For this review, take the finished solid that the model builds, in its own axes (mm). A direction names the side the tool comes from. Round coordinates to 2 decimals unless told otherwise and drop trailing zeros. Loops run counter-clockwise (first coordinate to the right, second up) from the corner with the lowest first, then second, coordinate; pieces in that order, holes last.
1) Mouldability with a two-part tool opening along Y and no side actions: class faces 4 (the flat face through (21.3, 4, 9)), 5 (the flat face through (29, 18, 6)), 6 (the flat face through (-3, -6, 5)), 7 (the flat face through (-3, 15, 1)) as pulls with the +Y half, pulls with the -Y half, needs draft (parallel to the pull), parting line crosses it, or undercut.
2) Tool access review of faces 1 (the flat face through (32.5, 3, 9)), 2 (the flat face through (23, 5, -2)), 3 (the flat face through (-5, 6, 5)): name each direction out of +Z, -Z, +X, -X, +Y, -Y from which nothing blocks a thin tool from reaching the whole face with its end or side.
3) Take a section at B-B (z = 8.75). State the section outline as (x, y) points.
4) Take a section at C-C (z = 4). State the section outline as (x, y) points, then the cut area to 3 significant figures.
5) Take a section at A-A (y = 7). State the section outline as (x, z) points (3 decimals), then the cut area to 3 significant figures.
6) Wall thickness on L1, parallel to X at y = 3.25, z = 0; L2, parallel to X at y = 15.5, z = 3.25; L3, parallel to Y at x = 32, z = 8.25: over which ranges is each line inside the solid? List them lowest first.
7) Take a section at D-D (y = 10). State the section outline as (x, z) points (3 decimals).
8) Insertion check: pin 1 (6 mm diameter, centred on x = 22.5, y = 4.5, fed in from -Z); pin 2 (0.5 mm diameter, centred on y = 2, z = 9, fed in from -X); pin 3 (4.5 mm diameter, centred on x = 36.5, z = -3, fed in from -Y); pin 4 (5.5 mm diameter, centred on x = 28, y = 6.5, fed in from +Z). Each pin has a flat end and moves straight along its axis. Give the tip position at first contact, or say it passes through.
Autodesk Fusion 360 part; units mm, degrees
sketch "Sketch1" plane through (0, 0, 0) normal (0, 1, 0) x (1, 0, 0)
  line L0 (0, 0) -> (25, 0)
  line L1 (25, 0) -> (25, -7)
  line L2 (25, -7) -> (1, -7)
  line L3 (0, -5) -> (0, 0)
  line L4 (-5, 5) -> (30, 5)
  line L5 (30, 5) -> (30, -10)
  line L6 (30, -10) -> (-5, -10)
  line L7 (-5, -10) -> (-5, 5)
  line L8 (1, -7) -> (1, -10)
  line L9 (-1, -5) -> (-1, -10)
  line L10 (0, -5) -> (-1, -5)
  dimension "d1" = 25
  dimension "d2" = 5
  dimension "d4" = 6
  dimension "d5" = 2
extrude "Extrude1" add sketch "Sketch1" along normal blind 18 contours L0 L1 L2 L3 L4 L5 L6 L7 L8 L9 L10 makes body 1
move_face "OffsetFaces1" offset -1 1 faces at (0, 6, 3.3333) on bodies 1
move_face "OffsetFaces2" offset 2 2 faces at (20.3333, 6, 10) (-2.3333, 6, 10) on bodies 1
extrude "Extrude2" cut 1 faces at (1, 6, 8.6667) along direction (1, 0, 0) blind 4 on bodies 1 bodies 1
split "Split1" by plane through (-1, 0, 5) normal (1, 0, 0) bodies 1 makes body 2 at (19.6667, 12, -5)
sketch "Sketch3" plane through (-1, 0, 0) normal (1, 0, 0) x (0, 1, 0)
  line L0 (18, -5) -> (18, 12)
  line L1 (18, 12) -> (0, 12)
  line L2 (0, 12) -> (0, -5)
  line L3 (0, -5) -> (18, -5)
  line L4 (18, 12) -> (0, 12)
  line L5 (0, 12) -> (0, 7)
  line L6 (0, 7) -> (18, 7)
  line L7 (18, 7) -> (18, 12)
extrude "Extrude3" add sketch "Sketch3" along normal blind 2 contours L0 L1 L2 L4 L5 L6 L7 bodies 1
combine "Combine1" operation add target body 1 tool bodies 2
sketch "Sketch4" plane through (0, 0, 0) normal (0, -1, 0) x (1, 0, 0)
  line L0 (1, 12) -> (-5, 12)
  line L1 (-5, 12) -> (-5, -5)
  line L2 (-5, -5) -> (30, -5)
  line L3 (30, -5) -> (30, 12)
  line L4 (30, 12) -> (5, 12)
  line L5 (5, 12) -> (5, 7)
  line L6 (5, 7) -> (25, 7)
  line L7 (25, 7) -> (25, 0)
  line L8 (25, 0) -> (-1, 0)
  line L9 (-1, 0) -> (-1, 7)
  line L10 (-1, 7) -> (1, 7)
  line L11 (1, 7) -> (1, 12)
  line L12 (23, -5) -> (23, 0)
  line L13 (17, -5) -> (17, 0)
  dimension "d14" = 7
  dimension "d15" = 6
extrude "Extrude4" cut sketch "Sketch4" against normal blind 9 contours L2 L8 L12 L13 bodies 1
sketch "Sketch5" plane through (0, 18, 0) normal (0, 1, 0) x (-1, 0, 0)
  line L0 (-30, -5) -> (5, -5)
  line L1 (5, -5) -> (5, 12)
  line L2 (5, 12) -> (-1, 12)
  line L3 (-1, 12) -> (-1, 7)
  line L4 (-1, 7) -> (1, 7)
  line L5 (1, 7) -> (1, 0)
  line L6 (1, 0) -> (-25, 0)
  line L7 (-25, 0) -> (-25, 7)
  line L8 (-25, 7) -> (-5, 7)
  line L9 (-5, 7) -> (-5, 12)
  line L10 (-5, 12) -> (-30, 12)
  line L11 (-30, 12) -> (-30, -5)
  line L12 (-30, 1) -> (5, 1)
  dimension "d18" = 6
extrude "Extrude5" cut sketch "Sketch5" against normal blind 6 contours L0 L1 L5 L6 L7 L11 L12 bodies 1
sketch "Sketch6" plane through (0, 0, 0) normal (0, -1, 0) x (1, 0, 0)
  line L0 (17, -5) -> (17, 0)
  line L1 (17, 0) -> (-1, 0)
  line L2 (-1, 0) -> (-1, 7)
  line L3 (-1, 7) -> (1, 7)
  line L4 (1, 7) -> (1, 12)
  line L5 (1, 12) -> (-5, 12)
  line L6 (-5, 12) -> (-5, -5)
  line L7 (-5, -5) -> (17, -5)
  line L8 (30, -5) -> (-5, -5)
  line L9 (-5, -5) -> (-5, 1)
  line L10 (-5, 1) -> (-1, 1)
  line L11 (-1, 1) -> (-1, 0)
  line L12 (-1, 0) -> (25, 0)
  line L13 (25, 0) -> (25, 1)
  line L14 (25, 1) -> (30, 1)
  line L15 (30, 1) -> (30, -5)
extrude "Extrude6" cut sketch "Sketch6" against normal blind 6 contours L0 L1 L2 L6 L7 L8 L9 L10 L11 L12 | L0 L8 L12 L13 L14 L15 bodies 1
extrude "Extrude7" add 2 faces at (20, 0, 10.3333) (-3.6667, 0, 6.6667) along direction (0, -1, 0) blind 6 on bodies 1 bodies 1
extrude "Extrude8" add 2 faces at (26, 6, -3.3333) (3.6667, 6, -3.3333) along direction (0, -1, 0) blind 5 on bodies 1 bodies 1
extrude "Extrude9" add 1 faces at (5, 7.3333, 0) along direction (0, 0, 1) blind 0.2 on bodies 1 bodies 1
extrude "Extrude10" add 2 faces at (-3.6667, -3.6667, 1) (26.6667, -3.6667, 1) along direction (0, 0, -1) blind 3 on bodies 1 bodies 1
extrude "Extrude11" add 1 faces at (5, 7.3333, 0.2) along direction (0, 0, 1) blind 0.5 on bodies 1 bodies 1
extrude "Extrude12" cut 2 faces at (26.6667, -3.6667, -2) (-3.6667, -3.6667, -2) along direction (0, 0, 1) blind 1 on bodies 1 bodies 1
extrude "Extrude13" add 1 faces at (30, 8, 8.3333) along direction (1, 0, 0) blind 10 on bodies 1 bodies 1
sketch "Sketch7" plane through (0, 0, 12) normal (0, 0, 1) x (-1, 0, 0)
  line L0 (-5, -18) -> (-5, 6)
  line L1 (-5, 6) -> (-40, 6)
  line L2 (-40, 6) -> (-40, -18)
  line L3 (-40, -18) -> (-5, -18)
  line L4 (-32.5, 5) -> (-32.5, -12.1)
  line L5 (-32.5, -12.1) -> (-21.3, -12.1)
  line L6 (-21.3, -12.1) -> (-21.3, 5)
  line L7 (-21.3, 5) -> (-32.5, 5)
  dimension "d40" = 11.2
  dimension "d41" = 17.1
  dimension "d42" = 7.5
  dimension "d43" = 1
extrude "Extrude14" cut sketch "Sketch7" against normal blind 0.7 contours L4 L5 L6 L7 bodies 1
extrude "Extrude15" cut 2 faces at (10.4333, 8.0333, 12) (-1, 2, 12) along direction (0, 0, -1) blind 1 on bodies 1 bodies 1
extrude "Extrude16" cut 1 faces at (25.0333, 0.7, 11.3) along direction (0, 0, -1) blind 1 on bodies 1 bodies 1
extrude "Extrude17" cut 2 faces at (10.4333, 8.0333, 11) (-1, 2, 11) along direction (0, 0, -1) blind 1.25 on bodies 1 bodies 1
extrude "Extrude18" cut 1 faces at (25.0333, 0.7, 10.3) along direction (0, 0, -1) blind 1.25 on bodies 1 bodies 1
extrude "Extrude19" add 1 faces at (20, 12, -3.1) along direction (0, 1, 0) blind 0.5 on bodies 1 bodies 1
extrude "Extrude20" cut 2 faces at (35, -3.6667, -1) (-3.6667, -3.6667, -1) along direction (0, 0, 1) blind 0.5 on bodies 1 bodies 1
sketch "Sketch8" plane through (40, 0, 0) normal (1, 0, 0) x (0, 1, 0)
  line L0 (1, -0.5) -> (1, -5)
  line L1 (1, -5) -> (12.5, -5)
  line L2 (12.5, -5) -> (12.5, 1)
  line L3 (12.5, 1) -> (18, 1)
  line L4 (18, 1) -> (18, 9.75)
  line L5 (18, 9.75) -> (-6, 9.75)
  line L6 (-6, 9.75) -> (-6, -0.5)
  line L7 (-6, -0.5) -> (1, -0.5)
  line L8 (18, 5.375) -> (-6, 5.375)
extrude "Extrude21" add sketch "Sketch8" along normal blind 22 contours L0 L1 L2 L3 L4 L6 L7 L8 bodies 1
extrude "Extrude22" cut 1 faces at (25.0333, 0.7, 9.05) along direction (0, 0, -1) blind 1 on bodies 1 bodies 1
extrude "Extrude23" cut 1 faces at (62, 8.6667, -1.5) along direction (-1, 0, 0) blind 8 on bodies 1 bodies 1
sketch "Sketch9" plane through (-5, 0, 0) normal (-1, 0, 0) x (0, -1, 0)
  line L0 (-1, -5) -> (-1, -0.5)
  line L1 (-1, -0.5) -> (6, -0.5)
  line L2 (6, -0.5) -> (6, 9.75)
  line L3 (6, 9.75) -> (-18, 9.75)
  line L4 (-18, 9.75) -> (-18, 1)
  line L5 (-18, 1) -> (-12.5, 1)
  line L6 (-12.5, 1) -> (-12.5, -5)
  line L7 (-12.5, -5) -> (-1, -5)
  line L8 (-12.5, 1) -> (6, 1)
extrude "Extrude24" add sketch "Sketch9" along normal blind 5 contours L0 L1 L2 L6 L7 L8 bodies 1
extrude "Extrude25" add 1 faces at (23, 12.5, -3.1) along direction (0, 1, 0) blind 1 on bodies 1 bodies 1
extrude "Extrude26" cut 1 faces at (54, 9.3333, -1.5) along direction (-1, 0, 0) blind 2.5 on bodies 1 bodies 1
extrude "Extrude27" cut 1 faces at (51.5, 9.3333, -1.5) along direction (-1, 0, 0) blind 0.5 on bodies 1 bodies 1
extrude "Extrude28" cut 1 faces at (22, 13.5, -3.1) along direction (0, -1, 0) blind 1 on bodies 1 bodies 1
extrude "Extrude29" cut 1 faces at (51, 8.6667, -1.5) along direction (-1, 0, 0) blind 5.75 on bodies 1 bodies 1
extrude "Extrude30" add 1 faces at (-10, 8.6667, -1.5) along direction (-1, 0, 0) blind 2 on bodies 1 bodies 1
equation "d40 = 10.70 mm + 0.5 mm"
equation "d41 = 16.20 mm + 0.9 mm"
Response:
1. face 4: undercut
1. face 5: pulls with the +Y half
1. face 6: pulls with the -Y half
1. face 7: needs draft
2. face 1: +Z
2. face 2: -Z, -Y
2. face 3: +Z, -X, +Y, -Y
3. outline: (-5, -6) - (1, -6) - (1, 18) - (-5, 18) - close; (5, -6) - (40, -6) - (40, 18) - (5, 18) - close; hole (21.3, -5) - (32.5, -5) - (32.5, 12.1) - (21.3, 12.1) - close
4. outline: (-5, -6) - (-1, -6) - (-1, 18) - (-5, 18) - close; (25, -6) - (45.25, -6) - (45.25, 18) - (25, 18) - close
4. area: 582 mm2
5. outline: (-12, -5) - (17, -5) - (17, 0.7) - (-1, 0.7) - (-1, 7) - (1, 7) - (1, 9.75) - (-5, 9.75) - (-5, 1) - (-12, 1) - close; (5, 7) - (25, 7) - (25, 0.7) - (23, 0.7) - (23, -5) - (45.25, -5) - (45.25, 5.375) - (40, 5.375) - (40, 9.75) - (32.5, 9.75) - (32.5, 8.05) - (21.3, 8.05) - (21.3, 9.75) - (5, 9.75) - close
5. area: 532 mm2
6. L1: x = -12 to 17, 23 to 45.25
6. L2: x = -5 to -1, 25 to 45.25
6. L3: y = -6 to -5, 12.1 to 18
7. outline: (-12, -5) - (45.25, -5) - (45.25, 5.375) - (40, 5.375) - (40, 9.75) - (32.5, 9.75) - (32.5, 8.05) - (21.3, 8.05) - (21.3, 9.75) - (5, 9.75) - (5, 7) - (25, 7) - (25, 0.7) - (-1, 0.7) - (-1, 7) - (1, 7) - (1, 9.75) - (-5, 9.75) - (-5, 1) - (-12, 1) - close
8. pin 1: stops at z = -5
8. pin 2: stops at x = -5
8. pin 3: stops at y = 1
8. pin 4: stops at z = 8.05
